Could you check a few things on this model? Use its own coordinates, in mm. A direction names the side the tool comes from. Give positions to 0.01 mm unless a question says otherwise; leave off trailing zeros. Loops run counter-clockwise (first coordinate to the right, second up) from the corner with the lowest first, then second, coordinate; pieces in that order, holes last. Notation, with made-up numbers: M 59.25,-33 L 101.25,-33 A19 cw 101.25,-3 Z; hole C 65.25,-0.75 d11. An arc over 180 degrees is marked long. Return JSON: item names as keys, results as strings. Group by question number.
1. If we mould it in two halves opening along Z, with no side actions, what happens to faces 4 (the flat face through (-31, 23, 30.5)), 5 (the cylindrical face through (6.542, 21.835, 35.521)), 6 (the flat face through (-31, -23, 14.5))? For each: +Z half, -Z half, draft (parallel to the pull), parting line (faces both ways), or undercut.
2. If we section it at B-B (x = -22): State how many separate pieces and enclosed holes the cut face has, plus the area to 3 significant figures.
3. Please list where these lines run through material, in increasing order: line 1 (Z direction, x = -36.55, y = 17.5); line 2 (Z direction, x = -31, y = -25.5); line 3 (Z direction, x = -32, y = -16).
4. For faces 1 (the cylindrical face through (34.995, -0.562, 16.762)), 2 (the cylindrical face through (37.995, -0.589, 19.283)), 3 (the flat face through (-32.044, -19.936, 21.12)), which set-ups out of +Z, -Z, +X, -X, +Y, -Y let a thin tool reach every point of the face, with its end or its side?
5. For pin 1 (7 mm diameter, centred on x = 27.5, y = 26.5, fed in from -Z); pin 2 (0.9 mm diameter, centred on y = -1, z = 35.5, fed in from -X); pin 3 (12 mm diameter, centred on x = -21, y = 5, fed in from -Z); pin 4 (3 mm diameter, centred on y = -17, z = 21.5, fed in from +X), each with a flat end and sliding along its axis, tell me the tip position at first contact or that it passes through.
6. If we section it at A-A (z = 17.5): Write out the boundary of the cut face in (x, y), plus the area to 3 significant figures.
```python
from build123d import *

# Parameters (mm, degrees)
SKETCH_W        = 76
SKETCH_H        = 76
SKETCH_R        = 35
SKETCH_R_2      = 1.7
PAD_DEPTH       = 34
SKETCH001_R     = 60
SKETCH001_R_2   = 38
POCKET_DEPTH    = 30
SKETCH002_R     = 38
PAD001_DEPTH    = 3
SKETCH003_W     = 100
SKETCH003_H     = 100
SKETCH003_W_2   = 80
SKETCH003_H_2   = 68
POCKET001_DEPTH = 37.001
SKETCH004_W     = 68
SKETCH004_H     = 16
PAD002_DEPTH    = 22
POCKET002_DEPTH = 25
POCKET003_DEPTH = 20
SKETCH030_R     = 35
POCKET004_DEPTH = 18
SKETCH031_R     = 1.7
POCKET005_DEPTH = 30
SKETCH022_R     = 1.7
SKETCH022_R_2   = 7
SKETCH022_W     = 3.5
SKETCH022_H     = 5
POCKET006_DEPTH = 5
SKETCH032_W     = 220
SKETCH032_H     = 220
POCKET007_DEPTH = 37.001
POCKET008_DEPTH = 20
FILLET_R        = 1.1
FILLET001_R     = 1.1
FILLET002_R     = 1.1
FILLET003_R     = 1.1
FILLET004_R     = 2
FILLET005_R     = 2
CHAMFER_SIZE    = 1.7
CHAMFER001_SIZE = 1.7
CHAMFER002_SIZE = 1.7
CHAMFER003_SIZE = 1.7
CHAMFER004_SIZE = 1.7
CHAMFER005_SIZE = 1.7
CHAMFER006_SIZE = 1.7
CHAMFER007_SIZE = 1.7


with BuildPart() as part:
    # Sketch → Pad (new body)
    with BuildSketch(Plane.XY):
        Rectangle(SKETCH_W, SKETCH_H)
        Circle(SKETCH_R, mode=Mode.SUBTRACT)
        with Locations((-30, 30)):
            Circle(SKETCH_R_2, mode=Mode.SUBTRACT)
        with Locations((30, 30)):
            Circle(SKETCH_R_2, mode=Mode.SUBTRACT)
        with Locations((30, -30)):
            Circle(SKETCH_R_2, mode=Mode.SUBTRACT)
        with Locations((-30, -30)):
            Circle(SKETCH_R_2, mode=Mode.SUBTRACT)
    extrude(amount=PAD_DEPTH)

    # Sketch001 → Pocket (cut)
    with BuildSketch(Plane.XY.offset(34)):
        Circle(SKETCH001_R)
        Circle(SKETCH001_R_2, mode=Mode.SUBTRACT)
    extrude(amount=-POCKET_DEPTH, mode=Mode.SUBTRACT)

    # Sketch002 → Pad001 (new body)
    with BuildSketch(Plane.XY.offset(34)):
        Circle(SKETCH002_R)
    extrude(amount=PAD001_DEPTH)

    # Sketch003 → Pocket001 (cut, through all)
    with BuildSketch(Plane.XY.offset(37)):
        Rectangle(SKETCH003_W, SKETCH003_H)
        Rectangle(SKETCH003_W_2, SKETCH003_H_2, mode=Mode.SUBTRACT)
    extrude(amount=-POCKET001_DEPTH, mode=Mode.SUBTRACT)

    # Sketch004 → Pad002 (new body)
    with BuildSketch(Plane(origin=(-38, 0, 0), x_dir=(0, -1, 0), z_dir=(-1, 0, 0))):
        with Locations((0, 22.5)):
            Rectangle(SKETCH004_W, SKETCH004_H)
    extrude(amount=-PAD002_DEPTH)

    # Sketch005 → Pocket002 (cut)
    with BuildSketch(Plane(origin=(0, 0, 14.5), x_dir=(1, 0, 0), z_dir=(0, 0, -1))):
        Polygon((-38, 23), (-38, -23), (-24, -34), (-55, -34), (-55, 34), (-24, 34), align=None)
    extrude(amount=-POCKET002_DEPTH, mode=Mode.SUBTRACT)

    # Sketch029 → Pocket003 (cut)
    with BuildSketch(Plane.YZ.offset(-16)):
        Polygon((-15.883419, 19.7), (-14.266838, 22.5), (-15.883419, 25.3), (-19.116581, 25.3), (-20.733162, 22.5), (-19.116581, 19.7), align=None)
        Polygon((14.266838, 22.5), (15.883419, 19.7), (19.116581, 19.7), (20.733162, 22.5), (19.116581, 25.3), (15.883419, 25.3), align=None)
    extrude(amount=-POCKET003_DEPTH, mode=Mode.SUBTRACT)

    # Sketch030 → Pocket004 (cut)
    with BuildSketch(Plane(origin=(0, 0, 14.5), x_dir=(1, 0, 0), z_dir=(0, 0, -1))):
        Circle(SKETCH030_R)
    extrude(amount=-POCKET004_DEPTH, mode=Mode.SUBTRACT)

    # Sketch031 → Pocket005 (cut)
    with BuildSketch(Plane(origin=(-38, 0, 0), x_dir=(0, -1, 0), z_dir=(-1, 0, 0))):
        with Locations((-17.5, 22.5)):
            Circle(SKETCH031_R)
        with Locations((17.5, 22.5)):
            Circle(SKETCH031_R)
        with BuildLine():
            ThreePointArc((-5, 29.5), (-12, 22.5), (-5, 15.5))
            Line((-5, 15.5), (5, 15.5))
            ThreePointArc((5, 15.5), (12, 22.5), (5, 29.5))
            Line((-5, 29.5), (5, 29.5))
        make_face()
    extrude(amount=-POCKET005_DEPTH, mode=Mode.SUBTRACT)

    # Sketch022 → Pocket006 (cut)
    with BuildSketch(Plane.XY.offset(37)):
        with Locations((0, 22)):
            Circle(SKETCH022_R)
        with Locations((0, -22)):
            Circle(SKETCH022_R)
        with Locations((-22, 0)):
            Circle(SKETCH022_R)
        with Locations((22, 0)):
            Circle(SKETCH022_R)
        Circle(SKETCH022_R_2)
        with Locations((-15, 0)):
            Circle(SKETCH022_R)
        with BuildLine():
            ThreePointArc((-23.660997, 14.014536), (-21.731705, 6.47943), (-14.196598, 8.408722))
            ThreePointArc((-8.408722, 14.196598), (-11.667262, 11.667262), (-14.196598, 8.408722))
            ThreePointArc((-8.408722, 14.196598), (-6.47943, 21.731705), (-14.014536, 23.660997))
            ThreePointArc((-14.014536, 23.660997), (-19.445436, 19.445436), (-23.660997, 14.014536))
        make_face()
        with BuildLine():
            ThreePointArc((8.408722, -14.196598), (11.667262, -11.667262), (14.196598, -8.408722))
            ThreePointArc((23.660997, -14.014536), (21.731705, -6.47943), (14.196598, -8.408722))
            ThreePointArc((14.014536, -23.660997), (19.445436, -19.445436), (23.660997, -14.014536))
            ThreePointArc((8.408722, -14.196598), (6.47943, -21.731705), (14.014536, -23.660997))
        make_face()
        with BuildLine():
            ThreePointArc((23.660997, 14.014536), (19.445436, 19.445436), (14.014536, 23.660997))
            ThreePointArc((14.014536, 23.660997), (6.47943, 21.731705), (8.408722, 14.196598))
            ThreePointArc((14.196598, 8.408722), (11.667262, 11.667262), (8.408722, 14.196598))
            ThreePointArc((14.196598, 8.408722), (21.731705, 6.47943), (23.660997, 14.014536))
        make_face()
        with BuildLine():
            ThreePointArc((-14.014536, -23.660997), (-6.47943, -21.731705), (-8.408722, -14.196598))
            ThreePointArc((-14.196598, -8.408722), (-11.667262, -11.667262), (-8.408722, -14.196598))
            ThreePointArc((-14.196598, -8.408722), (-21.731705, -6.47943), (-23.660997, -14.014536))
            ThreePointArc((-23.660997, -14.014536), (-19.445436, -19.445436), (-14.014536, -23.660997))
        make_face()
        with Locations((-10.25, 0)):
            Rectangle(SKETCH022_W, SKETCH022_H)
        with BuildLine():
            ThreePointArc((-27, 5), (-30, 8), (-33, 5))
            Line((-33, 5), (-33, -5))
            ThreePointArc((-33, -5), (-30, -8), (-27, -5))
            Line((-27, 5), (-27, -5))
        make_face()
        with BuildLine():
            ThreePointArc((33, 5), (30, 8), (27, 5))
            Line((27, 5), (27, -5))
            ThreePointArc((27, -5), (30, -8), (33, -5))
            Line((33, 5), (33, -5))
        make_face()
    extrude(amount=-POCKET006_DEPTH, mode=Mode.SUBTRACT)

    # Sketch032 → Pocket007 (cut, through all)
    with BuildSketch(Plane.XY.offset(37)):
        Rectangle(SKETCH032_W, SKETCH032_H)
        Polygon((-67.882251, 0), (0, 67.882251), (67.882251, 0), (0, -67.882251), align=None, mode=Mode.SUBTRACT)
    extrude(amount=-POCKET007_DEPTH, mode=Mode.SUBTRACT)

    # Sketch033 → Pocket008 (cut)
    with BuildSketch(Plane(origin=(33.941125, 33.941125, 0), x_dir=(-0.707107, 0.707107, 0), z_dir=(0.707107, 0.707107, 0))):
        with BuildLine():
            ThreePointArc((-4.5, 32), (-7.5, 29), (-4.5, 26))
            Line((-4.5, 26), (4.5, 26))
            ThreePointArc((4.5, 26), (7.5, 29), (4.5, 32))
            Line((-4.5, 32), (4.5, 32))
        make_face()
    extrude(amount=-POCKET008_DEPTH, mode=Mode.SUBTRACT)

    # Fillet
    fillet_edges = [part.edges().sort_by_distance(p)[0] for p in [
        (8.306624, 34, 23.5),
    ]]
    fillet(fillet_edges, radius=FILLET_R)

    # Fillet001
    fillet001_edges = [part.edges().sort_by_distance(p)[0] for p in [
        (-8.306624, 34, 23.5),
    ]]
    fillet(fillet001_edges, radius=FILLET001_R)

    # Fillet002
    fillet002_edges = [part.edges().sort_by_distance(p)[0] for p in [
        (-8.306624, -34, 7.25),
    ]]
    fillet(fillet002_edges, radius=FILLET002_R)

    # Fillet003
    fillet003_edges = [part.edges().sort_by_distance(p)[0] for p in [
        (8.306624, -34, 7.25),
    ]]
    fillet(fillet003_edges, radius=FILLET003_R)

    # Fillet004
    fillet004_edges = [part.edges().sort_by_distance(p)[0] for p in [
        (-32.317808, -19.98898, 37),
    ]]
    fillet(fillet004_edges, radius=FILLET004_R)

    # Fillet005
    fillet005_edges = [part.edges().sort_by_distance(p)[0] for p in [
        (32.317808, 19.98898, 37),
    ]]
    fillet(fillet005_edges, radius=FILLET005_R)

    # Chamfer
    chamfer_edges = [part.edges().sort_by_distance(p)[0] for p in [
        (-31.7, 30, 4),
    ]]
    chamfer(chamfer_edges, length=CHAMFER_SIZE)

    # Chamfer001
    chamfer001_edges = [part.edges().sort_by_distance(p)[0] for p in [
        (-31.7, -30, 4),
    ]]
    chamfer(chamfer001_edges, length=CHAMFER001_SIZE)

    # Chamfer002
    chamfer002_edges = [part.edges().sort_by_distance(p)[0] for p in [
        (28.3, 30, 4),
    ]]
    chamfer(chamfer002_edges, length=CHAMFER002_SIZE)

    # Chamfer003
    chamfer003_edges = [part.edges().sort_by_distance(p)[0] for p in [
        (28.3, -30, 4),
    ]]
    chamfer(chamfer003_edges, length=CHAMFER003_SIZE)

    # Chamfer004
    chamfer004_edges = [part.edges().sort_by_distance(p)[0] for p in [
        (-23.7, 0, 37),
    ]]
    chamfer(chamfer004_edges, length=CHAMFER004_SIZE)

    # Chamfer005
    chamfer005_edges = [part.edges().sort_by_distance(p)[0] for p in [
        (-1.7, -22, 37),
    ]]
    chamfer(chamfer005_edges, length=CHAMFER005_SIZE)

    # Chamfer006
    chamfer006_edges = [part.edges().sort_by_distance(p)[0] for p in [
        (20.3, 0, 37),
    ]]
    chamfer(chamfer006_edges, length=CHAMFER006_SIZE)

    # Chamfer007
    chamfer007_edges = [part.edges().sort_by_distance(p)[0] for p in [
        (-1.7, 22, 37),
    ]]
    chamfer(chamfer007_edges, length=CHAMFER007_SIZE)


solid = part.part
```
Answer:
{
 "1": {"face 4": "+Z half", "face 5": "draft", "face 6": "undercut"},
 "2": {"separate pieces": "4", "enclosed holes": "0", "area": "488 mm²"},
 "3": {"line 1": "z = 0 to 4, 14.5 to 20.8, 24.2 to 30.5", "line 2": "z = 0 to 4, 14.5 to 30.5", "line 3": "z = 0 to 19.7, 25.3 to 37"},
 "4": {"face 1": "-Z", "face 2": "+Z, +X", "face 3": "none"},
 "5": {"pin 1": "stops at z = 0", "pin 2": "stops at x = -37.99", "pin 3": "stops at z = 34", "pin 4": "stops at x = 34.7"},
 "6": {"outline": "M -38,-23 L -24,-34 L -14.86,-34 A1.1 ccw -14.41,-31.9 A35 cw -33.57,-9.9 L -38,-9.9 Z; M -38,9.9 L -33.57,9.9 A35 cw -14.41,31.9 A1.1 ccw -14.86,34 L -24,34 L -38,23 Z; M 14.41,-31.9 A1.1 ccw 14.86,-34 L 16.97,-34 A38 ccw 16.97,34 L 14.86,34 A1.1 ccw 14.41,31.9 A35 cw Z", "area": "692 mm²"}
}
